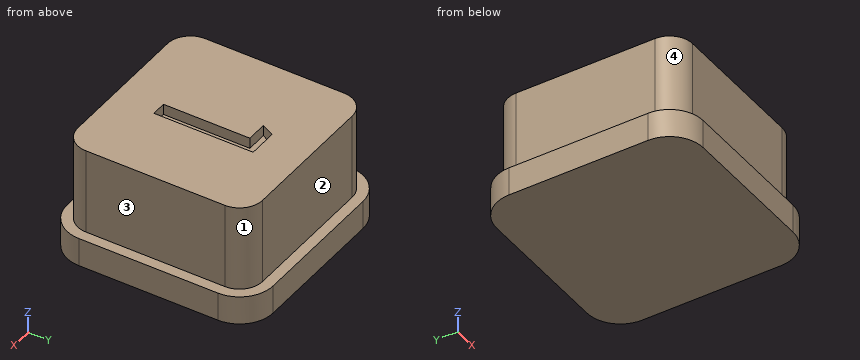
```python
from build123d import *

# Parameters (mm, degrees)
F1_DEPTH = 2
F2_DEPTH = 8
F3_DEPTH = 7.25


with BuildPart() as f1:
    # F0 (on Top) → F1 (new body)
    with BuildSketch(Plane.XY):
        with BuildLine():
            Line((4.85, 7.2), (-4.85, 7.2))
            ThreePointArc((-4.85, 7.2), (-6.511701, 6.511701), (-7.2, 4.85))
            Line((-7.2, 4.85), (-7.2, -4.85))
            ThreePointArc((-7.2, -4.85), (-6.511701, -6.511701), (-4.85, -7.2))
            Line((-4.85, -7.2), (4.85, -7.2))
            ThreePointArc((4.85, -7.2), (6.511701, -6.511701), (7.2, -4.85))
            Line((7.2, -4.85), (7.2, 4.85))
            ThreePointArc((7.2, 4.85), (6.511701, 6.511701), (4.85, 7.2))
        make_face()
        with BuildLine():
            ThreePointArc((6.45, -4.85), (5.981371, -5.981371), (4.85, -6.45))
            Line((4.85, -6.45), (-4.85, -6.45))
            ThreePointArc((-4.85, -6.45), (-5.981371, -5.981371), (-6.45, -4.85))
            Line((-6.45, -4.85), (-6.45, 4.85))
            ThreePointArc((-6.45, 4.85), (-5.981371, 5.981371), (-4.85, 6.45))
            Line((-4.85, 6.45), (4.85, 6.45))
            ThreePointArc((4.85, 6.45), (5.981371, 5.981371), (6.45, 4.85))
            Line((6.45, 4.85), (6.45, -4.85))
        make_face(mode=Mode.SUBTRACT)
    extrude(amount=F1_DEPTH)

    # F0 (on Top) → F2 (join)
    with BuildSketch(Plane.XY):
        with BuildLine():
            Line((-4.85, -6.45), (4.85, -6.45))
            ThreePointArc((4.85, -6.45), (5.981371, -5.981371), (6.45, -4.85))
            Line((6.45, -4.85), (6.45, 4.85))
            ThreePointArc((6.45, 4.85), (5.981371, 5.981371), (4.85, 6.45))
            Line((4.85, 6.45), (-4.85, 6.45))
            ThreePointArc((-4.85, 6.45), (-5.981371, 5.981371), (-6.45, 4.85))
            Line((-6.45, 4.85), (-6.45, -4.85))
            ThreePointArc((-6.45, -4.85), (-5.981371, -5.981371), (-4.85, -6.45))
        make_face()
        Polygon((1.243107, -3.466724), (0.205538, -3.466724), (0.205538, 2.567429), (-1.243232, 2.567429), (-0.803342, 3.466336), (1.243107, 3.466336), align=None, mode=Mode.SUBTRACT)
    extrude(amount=F2_DEPTH)

    # F0 (on Top) → F3 (join)
    with BuildSketch(Plane.XY):
        Polygon((0.205538, 2.567429), (0.205538, -3.466724), (1.243107, -3.466724), (1.243107, 3.466336), (-0.803342, 3.466336), (-1.243232, 2.567429), align=None)
    extrude(amount=F3_DEPTH)


solid = f1.part
```
Source: CAD feature listing. Evaluate the final solid. Frame: model axes, mm. Face numbers are marked on the shaded views. A direction names the side the tool comes from. Give positions to 0.01 mm unless a question says otherwise; leave off trailing zeros. Order: outer loops, then holes, each group sorted by start corner. A loop starts at its lowest first (then second) coordinate and runs counter-clockwise, first axis right, second up. Notation, with made-up numbers: (36, -37) -> (73, -37) arc R28 ccw to (73, -17) -> close; hole circle Ø3 at (60.25, 26). An arc over 180 degrees is marked (long way). Use a Markdown table: item, result.
Q1. Section A-A (y = -1.25). Return the cut outline in (x, z).
A:
| item | result |
|---|---|
| outline | (-7.2, 0) -> (7.2, 0) -> (7.2, 2) -> (6.45, 2) -> (6.45, 8) -> (1.24, 8) -> (1.24, 7.25) -> (0.21, 7.25) -> (0.21, 8) -> (-6.45, 8) -> (-6.45, 2) -> (-7.2, 2) -> close |
Q2. Section D-D (y = 4.5). Return the cut outline in (x, z).
A:
| item | result |
|---|---|
| outline | (-7.2, 0) -> (7.2, 0) -> (7.2, 2) -> (6.45, 2) -> (6.45, 8) -> (-6.45, 8) -> (-6.45, 2) -> (-7.2, 2) -> close |
Q3. Section C-C (z = 0.75). Return the cut outline in (x, y).
A:
| item | result |
|---|---|
| outline | (-7.2, -4.85) arc R2.35 ccw to (-4.85, -7.2) -> (4.85, -7.2) arc R2.35 ccw to (7.2, -4.85) -> (7.2, 4.85) arc R2.35 ccw to (4.85, 7.2) -> (-4.85, 7.2) arc R2.35 ccw to (-7.2, 4.85) -> close |
Q4. Section B-B (x = 1). Return the cut outline in (y, z), and give its area (3 significant figures).
A:
| item | result |
|---|---|
| outline | (-7.2, 0) -> (7.2, 0) -> (7.2, 2) -> (6.45, 2) -> (6.45, 8) -> (3.47, 8) -> (3.47, 7.25) -> (-3.47, 7.25) -> (-3.47, 8) -> (-6.45, 8) -> (-6.45, 2) -> (-7.2, 2) -> close |
| area | 101 mm^2 |
Q5. Material intervals for line 1 (Y direction, x = 1.5, z = 6.5); line 2 (Z direction, x = 5.25, y = -6.5), sorted ascending. Write a range as [from, to].
A:
| item | result |
|---|---|
| line 1 | [-6.45, 6.45] |
| line 2 | [0, 2] |
Q6. First-contact query: P1, Ø1.8, axis at y = -1, z = 3.5, coming from the -X side; P2, Ø0.6, axis at x = 0.5, z = 7.5, coming from the -Y side; P3, Ø0.6, axis at x = 0, z = 7.5, coming from the +Y side. Flat tips, straight axial feed; report the tip coordinate or a pass-through.
A:
| item | result |
|---|---|
| P1 | x = -6.45 |
| P2 | y = -6.45 |
| P3 | y = 6.45 |
Q7. Access query for the marked faces 1, 2, 3 and 4. Directions: +Z, -Z, +X, -X, +Y, -Y. A direction counts if a zero-diameter tool reaches every point of the face in a straight line with its end or side. Return the directions, or none.
A:
| item | result |
|---|---|
| face 1 | +Z, +X, +Y |
| face 2 | +Z, +X, -X, +Y |
| face 3 | +Z, +X, +Y, -Y |
| face 4 | +Z, -X, -Y |
